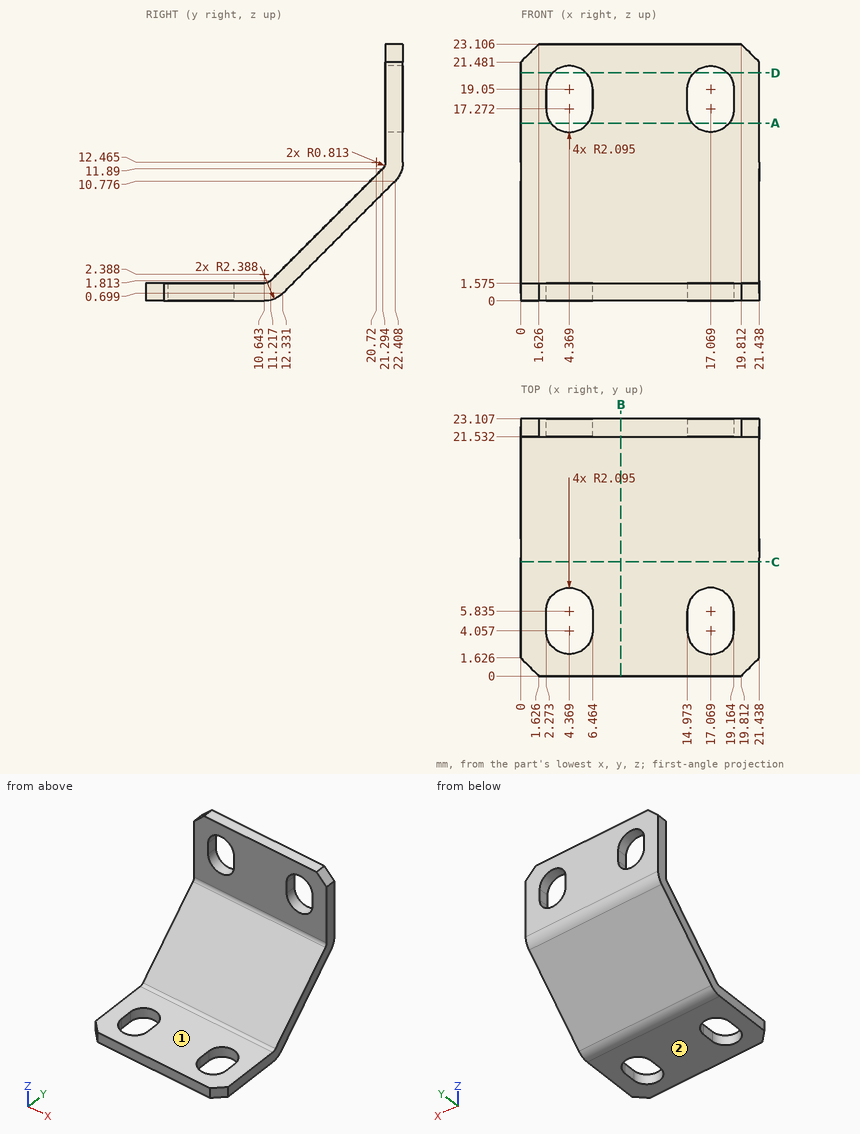
Check sheet for the drawn part. Datum: minimum x, y, z corner. Units: mm. A direction names the side the tool comes from. Round coordinates to 2 decimals unless told otherwise and drop trailing zeros. Order: outer loops, then holes, each group sorted by start corner. A loop starts at its lowest first (then second) coordinate and runs counter-clockwise, first axis right, second up.
1. Section check D-D on z = 20.5. Record the cut outline in (x, y) (1 decimal).
Final values:
outline: (0, 21.5) - (2.9, 21.5) - (2.9, 23.1) - (0, 23.1) - close; (5.9, 21.5) - (15.6, 21.5) - (15.6, 23.1) - (5.9, 23.1) - close; (18.6, 21.5) - (21.4, 21.5) - (21.4, 23.1) - (18.6, 23.1) - close
2. Thickness scan on L1, parallel to Z at x = 20, y = 3.25 (1 decimal); L2, parallel to Y at x = 3.5, z = 5.25 (1 decimal); L3, parallel to Z at x = 16.25, y = 19 (1 decimal). Record the ranges inside material, lowest first.
Final values:
L1: z = 0 to 1.6
L2: y = 14.7 to 16.9
L3: z = 7.4 to 9.6
3. Go/stop test with flat-tipped pins: P1, Ø1, axis at x = 12, z = 18.5, coming from the -Y side; P2, Ø3, axis at x = 18.5, z = 10.5, coming from the -Y side (1 decimal); P3, Ø3, axis at x = 8, y = 7.5, coming from the +Z side (1 decimal). Record where each tip stops, or that it passes through.
Final values:
P1: stops at y = 21.53
P2: stops at y = 18.4
P3: stops at z = 1.6
4. Access from +Z, -Z, +X, -X, +Y, -Y to the whole of each face (thin tool, end or side, straight path). Record for the marked faces 1 and 2.
Final values:
face 1: +Z, +X, -X, -Y
face 2: -Z, +X, -X, +Y, -Y
5. Section check B-B on x = 9. Record the cut outline in (y, z) (1 decimal).
Final values:
outline: (0, 0) - (10.6, 0) arc R2.4 ccw to (12.3, 0.7) - (22.4, 10.8) arc R2.4 ccw to (23.1, 12.5) - (23.1, 23.1) - (21.5, 23.1) - (21.5, 12.5) arc R0.8 cw to (21.3, 11.9) - (11.2, 1.8) arc R0.8 cw to (10.6, 1.6) - (0, 1.6) - close
6. Section check C-C on y = 10.25. Record the cut outline in (x, z) (1 decimal).
Final values:
outline: (0, 0) - (21.4, 0) - (21.4, 1.6) - (0, 1.6) - close
7. Section check A-A on z = 16. Record the cut outline in (x, y) (1 decimal).
Final values:
outline: (0, 21.5) - (2.7, 21.5) - (2.7, 23.1) - (0, 23.1) - close; (6, 21.5) - (15.4, 21.5) - (15.4, 23.1) - (6, 23.1) - close; (18.7, 21.5) - (21.4, 21.5) - (21.4, 23.1) - (18.7, 23.1) - close
